from build123d import *

# Parameters (mm, degrees)
EXTRUDE_1_DEPTH = 10
FILLET_1_R      = 0.2


with BuildPart() as part:
    # Эскиз1 → Бобышка-Вытянуть1 (new body, symmetric)
    with BuildSketch(Plane.XY):
        Polygon((4, 0), (-4, 0), (-4, -3.3), (-9.75, -3.3), (-9.75, -5.8), (-4, -9.5), (4, -9.5), (9.75, -5.8), (9.75, -3.3), (4, -3.3), align=None)
    extrude(amount=EXTRUDE_1_DEPTH, both=True)

    # Эскиз4 → Отверстие обработанное метчиком M63 (revolve, cut)
    with BuildSketch(Plane(origin=(0, 0, 0), x_dir=(0, 0, 1), z_dir=(1, 0, 0))):
        Polygon((0, 0), (0, 9.5), (3.025, 9.5), (2.5, 8.975), (2.5, 0.525), (3.025, 0), align=None)
    revolve(axis=Axis((0, 6.35, 0), (0, -1, 0)), mode=Mode.SUBTRACT)

    # Скругление1
    fillet_1_edges = [part.edges().sort_by_distance(p)[0] for p in [
        (-4, 0, 0),
        (4, 0, 0),
        (4, -3.3, 0),
        (9.75, -3.3, 0),
        (4, -9.5, 0),
        (-4, -9.5, 0),
        (-9.75, -3.3, 0),
        (-4, -3.3, 0),
    ]]
    fillet(fillet_1_edges, radius=FILLET_1_R)


solid = part.part
Model file for the job. Use its own axes, mm. A direction names the side the tool comes from. Give positions to 0.01 mm unless a question says otherwise; leave off trailing zeros. Loops run counter-clockwise (first coordinate to the right, second up) from the corner with the lowest first, then second, coordinate; pieces in that order, holes last. Notation, with made-up numbers: (-36, -18) -> (21, -18) arc R15 cw to (21, 3) -> close; hole circle Ø11 at (-1, -18). An arc over 180 degrees is marked (long way). Use a Markdown table: item, result. Add a question column.
(1) Slice it at B-B on x = 0. List the corners of the cut face in (y, z) (3 decimals).
(2) Slice it at A-A on z = 0. List the corners of the cut face in (x, y) (3 decimals), and give its area (3 significant figures).
(3) Drop flat-ended pins along their axis: pin 1 Ø3 at (y, z) = (-1.5, 2.5) entering from -X; pin 2 Ø1.5 at (x, z) = (5, 5) entering from -Y; pin 3 Ø4.5 at (x, z) = (6.5, 4.5) entering from +Y. Give the stop position or say it passes through.
(4) Mould opens along X. For faces 4 (the cylindrical face through (2.44, -4.69, -0.54)), 5 (the flat face through (4, -2, 0)), 6 (the flat face through (0, -5, -10)) say: +X half, -X half, draft (parallel to the pull), parting line (faces both ways), or undercut.
(5) Slice it at D-D on z = 5.5. List the corners of the cut face in (x, y), and give its area (3 significant figures).
(6) Wall check: line 1 along X through (y, z) = (-3.5, 0); line 2 along Z through (x, y) = (0, -6). Give the ranges that are in metal, low to high.
(7) Tool access for faces 1 (the flat face through (7, -3.3, 0)), 2 (the flat face through (-7, -3.3, 0)), 3 (the flat face through (-3, -9.5, -2)): list every direction of +Z, -Z, +X, -X, +Y, -Y with a clear straight run to the whole face (end or side of a thin tool).
(8) Slice it at C-C on y = -2.25. List the corners of the cut face in (x, z).
Filled sheet:
| question | item | result |
|---|---|---|
| 1 | outline | (-9.5, -10) -> (0, -10) -> (0, -3.025) -> (-0.525, -2.5) -> (-8.975, -2.5) -> (-9.5, -3.025) -> close; (-9.5, 3.025) -> (-8.975, 2.5) -> (-0.525, 2.5) -> (0, 3.025) -> (0, 10) -> (-9.5, 10) -> close |
| 2 | outline | (-9.75, -5.8) -> (-4.049, -9.468) arc R0.2 ccw to (-3.941, -9.5) -> (-3.025, -9.5) -> (-2.5, -8.975) -> (-2.5, -0.525) -> (-3.025, 0) -> (-3.8, 0) arc R0.2 ccw to (-4, -0.2) -> (-4, -3.1) arc R0.2 cw to (-4.2, -3.3) -> (-9.55, -3.3) arc R0.2 ccw to (-9.75, -3.5) -> close; (2.5, -8.975) -> (3.025, -9.5) -> (3.941, -9.5) arc R0.2 ccw to (4.049, -9.468) -> (9.75, -5.8) -> (9.75, -3.5) arc R0.2 ccw to (9.55, -3.3) -> (4.2, -3.3) arc R0.2 cw to (4, -3.1) -> (4, -0.2) arc R0.2 ccw to (3.8, 0) -> (3.025, 0) -> (2.5, -0.525) -> close |
| 2 | area | 78.0 mm2 |
| 3 | pin 1 | x = -4 |
| 3 | pin 2 | y = -9.34 |
| 3 | pin 3 | y = -3.3 |
| 4 | face 4 | undercut |
| 4 | face 5 | +X half |
| 4 | face 6 | draft |
| 5 | outline | (-9.75, -5.8) -> (-4.05, -9.47) arc R0.2 ccw to (-3.94, -9.5) -> (3.94, -9.5) arc R0.2 ccw to (4.05, -9.47) -> (9.75, -5.8) -> (9.75, -3.5) arc R0.2 ccw to (9.55, -3.3) -> (4.2, -3.3) arc R0.2 cw to (4, -3.1) -> (4, -0.2) arc R0.2 ccw to (3.8, 0) -> (-3.8, 0) arc R0.2 ccw to (-4, -0.2) -> (-4, -3.1) arc R0.2 cw to (-4.2, -3.3) -> (-9.55, -3.3) arc R0.2 ccw to (-9.75, -3.5) -> close |
| 5 | area | 126 mm2 |
| 6 | line 1 | -9.75 to -2.5, 2.5 to 9.75 |
| 6 | line 2 | -10 to -2.5, 2.5 to 10 |
| 7 | face 1 | +Z, -Z, +X, +Y |
| 7 | face 2 | +Z, -Z, -X, +Y |
| 7 | face 3 | +Z, -Z, +X, -X, -Y |
| 8 | outline | (-4, -10) -> (4, -10) -> (4, 10) -> (-4, 10) -> close; hole circle Ø5 at (0, 0) |
